Could you check a few things on this model? Use its own coordinates, in mm. Round coordinates to 2 decimals unless told otherwise and drop trailing zeros. Write each loop counter-clockwise with the first axis right and the second up, starting at its lowest first coordinate (ties: lowest second). Pieces come first, ordered by that corner, then holes. Notation, with made-up numbers: (-27, 5) - (8, 5) arc R20 ccw to (8, 37) - close; hole circle Ø2 at (-13, 48). An arc over 180 degrees is marked (long way). Put each result on its own line as item: value.
from build123d import *

# Parameters (mm, degrees)
SKETCH1_R           = 5.5
BOSS_EXTRUDE1_DEPTH = 30.1
SKETCH2_R           = 3
CUT_EXTRUDE1_DEPTH  = 31.1
FILLET1_R           = 0.5


with BuildPart() as part:
    # Sketch1 → Boss-Extrude1 (new body)
    with BuildSketch(Plane.XY):
        Circle(SKETCH1_R)
    extrude(amount=BOSS_EXTRUDE1_DEPTH)

    # Sketch2 → Cut-Extrude1 (cut, through all)
    with BuildSketch(Plane.XY.offset(30.1)):
        Circle(SKETCH2_R)
    extrude(amount=-CUT_EXTRUDE1_DEPTH, mode=Mode.SUBTRACT)

    # Fillet1
    fillet1_edges = [part.edges().sort_by_distance(p)[0] for p in [
        (-5.5, 0, 0),
        (-5.5, 0, 30.1),
        (-3, 0, 0),
        (-3, 0, 30.1),
    ]]
    fillet(fillet1_edges, radius=FILLET1_R)


solid = part.part
(1) Please list where these lines run through material, in increasing order: probe 1 along Z at (x, y) = (-0.75, 5); probe 2 along X at (y, z) = (1.75, 21); probe 3 along Y at (x, z) = (1.25, 19). Write a range as from..to.
Values found:
probe 1: z = 0..30.1
probe 2: x = -5.21..-2.44, 2.44..5.21
probe 3: y = -5.36..-2.73, 2.73..5.36
(2) I'm going to push flat-ended pins straight in: pin 1 (2 mm diameter, centred on x = 1.5, z = 10, fed in from +Y); pin 2 (2 mm diameter, centred on x = -1.5, z = 15.5, fed in from -Y); pin 3 (4 mm diameter, centred on y = -4, z = 27, fed in from +X). Where does each tip first touch, or does it pass through?
Values found:
pin 1: stops at y = 5.48
pin 2: stops at y = -5.48
pin 3: stops at x = 5.12
(3) Imagine slicing it at C-C, the plane z = 21. List the corners of the cut face in (x, y) for me, then the cut area to 3 significant figures.
Values found:
outline: circle Ø11 at (0, 0); hole circle Ø6 at (0, 0)
area: 66.8 mm^2
(4) Imagine slicing it at A-A, the plane y = 0. List the corners of the cut face in (x, z) for me, then the cut area to 3 significant figures.
Values found:
outline: (-5.5, 0.5) arc R0.5 ccw to (-5, 0) - (-3.5, 0) arc R0.5 ccw to (-3, 0.5) - (-3, 29.6) arc R0.5 ccw to (-3.5, 30.1) - (-5, 30.1) arc R0.5 ccw to (-5.5, 29.6) - close; (3, 0.5) arc R0.5 ccw to (3.5, 0) - (5, 0) arc R0.5 ccw to (5.5, 0.5) - (5.5, 29.6) arc R0.5 ccw to (5, 30.1) - (3.5, 30.1) arc R0.5 ccw to (3, 29.6) - close
area: 150 mm^2
(5) If we mould it in two halves opening along X, with no side actions, what happens to faces 1 (the face through (2.2, -3.3, 0)), 2 (the face through (-1.19, -5.37, 14.85)), 3 (the face through (-3, 0, 15))? For each: pulls with the +X half, pulls with the -X half, needs draft (parallel to the pull), parting line crosses it, or undercut.
Values found:
face 1: needs draft
face 2: parting line crosses it
face 3: undercut
